Autodesk Inventor part; units mm, degrees
ref_plane "YZ Plane" through (0, 0, 0) normal (1, 0, 0) x (0, 1, 0)
ref_plane "XZ Plane" through (0, 0, 0) normal (0, 1, 0) x (-1, 0, 0)
ref_plane "XY Plane" through (0, 0, 0) normal (0, 0, 1) x (1, 0, 0)
sketch "Sketch1" plane through (0, 0, 0) normal (1, 0, 0) x (0, 1, 0)
  line L0 (0, 0) -> (1.7, 0) construction
  line L1 (1.7, 0) -> (4.95, 0)
  line L2 (4.95, 0) -> (4.95, -1.5)
  line L3 (4.95, -1.5) -> (3.95, -1.5)
  line L4 (3.95, -1.5) -> (3.95, -5)
  line L5 (3.95, -5) -> (1.7, -5)
  line L6 (1.7, -5) -> (1.7, 0)
  line L7 (0, 0) -> (0, -13.7466) construction
  dimension "d0" = 1.7
  dimension "d1" = 3.95
  dimension "d2" = 1
  dimension "d3" = 1.5
  dimension "d4" = 3.5
revolve "Revolution1" add sketch "Sketch1" angle 360 about axis through (0, 0, 0) along (0, 0, -1)
sketch "Sketch2" plane through (0, 0, 0) normal (0, 0, 1) x (1, 0, 0)
  line L0 (2.85, -2.85) -> (-2.85, -2.85)
  line L1 (-2.85, -2.85) -> (-2.85, 2.85)
  line L2 (-2.85, 2.85) -> (2.85, 2.85)
  line L3 (2.85, 2.85) -> (2.85, -2.85)
  line L4 (2.85, -2.85) -> (-2.85, 2.85) construction
  line L5 (-2.85, -2.85) -> (2.85, 2.85) construction
  point P0 (0, 0)
  dimension "d6" = 5.7
extrude "Extrusion1" cut sketch "Sketch2" against normal blind 2.7
fillet "Fillet1" radius 0.5 2 edges at (0, -3.95, -5) (0, -1.7, -5)
sketch "Sketch3" plane through (0, 0, -2.7) normal (0, 0, 1) x (1, 0, 0)
  line L0 (-2.85, 2.85) -> (2.85, 2.85)
  line L1 (2.735, -2.85) -> (-2.735, -2.85)
  line L2 (-1.7, 2.85) -> (1.7, 2.85)
  line L3 (1.7, 2.85) -> (1.7, -2.85)
  line L4 (1.7, -2.85) -> (-1.7, -2.85)
  line L5 (-1.7, -2.85) -> (-1.7, 2.85)
  arc A0 (-2.85, -2.735) -> (-2.735, -2.85) centre (0, 0) ccw
  line L6 (2.735, -2.85) -> (-2.735, -2.85)
  arc A1 (2.735, -2.85) -> (2.85, -2.735) centre (0, 0) ccw
  line L7 (2.85, 2.735) -> (2.85, -2.735)
  arc A2 (2.85, 2.735) -> (2.735, 2.85) centre (0, 0) ccw
  line L8 (-2.735, 2.85) -> (2.735, 2.85)
  arc A3 (-2.735, 2.85) -> (-2.85, 2.735) centre (0, 0) ccw
  line L9 (-2.85, -2.735) -> (-2.85, 2.735)
  circle A4 centre (0, 0) radius 1.7
  point P0 (-1.7, 0)
  point P1 (1.7, 0)
  point P2 (1.7, 2.85)
extrude "Extrusion2" cut sketch "Sketch3" against normal blind 0.2 contours L0 L3 A4 L5 | A4 L3 L1 L5
properties part number "HD_BearingShaft1"
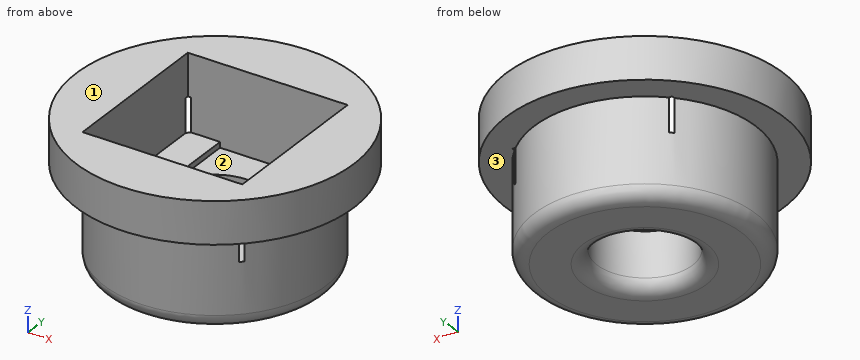
For this review, take the finished solid that the model builds, in its own axes (mm). Face numbers are marked on the shaded views. A direction names the side the tool comes from. Give positions to 0.01 mm unless a question says otherwise; leave off trailing zeros. Order: outer loops, then holes, each group sorted by start corner. A loop starts at its lowest first (then second) coordinate and runs counter-clockwise, first axis right, second up. Notation, with made-up numbers: (42, 34) - (100, 34) arc R6 cw to (100, 44) - close; hole circle Ø9 at (42.25, 66). An arc over 180 degrees is marked (long way). Answer as a JSON object with one key per item and string values. Group by question number.
Item 1: Take a section at A-A on x = 0. Give the boundary of the cut face in (y, z), and give its area (3 significant figures).
Item 2: Clearance check with flat-ended pins moving along their axes: pin 1 Ø1.3 at (x, y) = (2, -1) entering from +Z; pin 2 Ø1.5 at (y, z) = (4, -4) entering from +X (3 decimals); pin 3 Ø0.9 at (x, y) = (-0.5, 1) entering from +Z. State where each tip first meets the part, or that it passes through.
Item 3: Machinability: for the marked faces 1, 2 and 3, which of the approach directions +Z, -Z, +X, -X, +Y, -Y give a long, thin tool a straight path to every point of the face, cutting with its end or side? Answer none if there is none.
Item 4: Wall thickness on line 1 along X through (y, z) = (0, -3.55); line 2 along Y through (x, z) = (-1, -0.4): over which ranges is each line inside the solid? List them lowest first.
Reported:
{
 "1": {"outline": "(-4.95, -1.5) - (-3.95, -1.5) - (-3.95, -4.5) arc R0.5 ccw to (-3.45, -5) - (-2.2, -5) arc R0.5 ccw to (-1.7, -4.5) - (-1.7, -2.9) - (-2.85, -2.9) - (-2.85, 0) - (-4.95, 0) - close; (1.7, -4.5) arc R0.5 ccw to (2.2, -5) - (3.45, -5) arc R0.5 ccw to (3.95, -4.5) - (3.95, -1.5) - (4.95, -1.5) - (4.95, 0) - (2.85, 0) - (2.85, -2.9) - (1.7, -2.9) - close", "area": "18.6 mm^2"},
 "2": {"pin 1": "z = -2.7", "pin 2": "x = 2.245", "pin 3": "through"},
 "3": {"face 1": "+Z, +X, -X, +Y, -Y", "face 2": "+Z", "face 3": "-Z"},
 "4": {"line 1": "-3.95 to -1.7, 1.7 to 3.95", "line 2": "-4.85 to -2.85, 2.85 to 4.85"}
}
